from build123d import *

# Parameters (mm, degrees)
F1_DEPTH = 46
F2_R     = 1
F3_DEPTH = 20.001
F5_D     = 4


with BuildPart() as f1:
    # F0 (on Front) → F1 (new body)
    with BuildSketch(Plane.XZ):
        Polygon((33, 0), (0, 0), (0, -20), (7, -20), (7, -7), (33, -7), align=None)
    extrude(amount=F1_DEPTH)

    # F2 (on face) → F3 (cut, through all)
    with BuildSketch(Plane.XY):
        with Locations((24, -4.5)):
            Circle(F2_R)
        with Locations((24, -41.5)):
            Circle(F2_R)
    extrude(amount=-F3_DEPTH, mode=Mode.SUBTRACT)

    # F5 (through all)
    with Locations(Plane.YZ.offset(7)):
        with Locations((-41.5, -13.5), (-4.5, -13.5)):
            Hole(F5_D / 2)


solid = f1.part
Can you work these out from the model? Positions are in its coordinate system, mm. A direction names the side the tool comes from. Coordinates: 2 decimals unless noted, no trailing zeros. Loops run counter-clockwise (first coordinate to the right, second up) from the corner with the lowest first, then second, coordinate; pieces in that order, holes last. Notation, with made-up numbers: M 40,33 L 77,33 A33 cw 77,62 Z; hole C 61,13 d4. An arc over 180 degrees is marked long. Answer as CSV lines item,"result". Start each with the question number.
1. Suppose I cut it at D-D, the plane y = -11.5. List the corners of the cut face in (x, z) for me.
2. For pin 1 Ø8 at (x, y) = (17, -17.5) entering from -Z; pin 2 Ø1 at (y, z) = (-7.5, -17) entering from +X, each with a flat end and sliding along its axis, tell me the tip position at first contact or that it passes through.
3. If I drill on probe 1 along Y at (x, z) = (24, -2); probe 2 along X at (y, z) = (-7.5, -18); probe 3 along Z at (x, y) = (10.5, -26.5), over which ranges is the centre line in solid material (lowest first)? Write a range as [from, to].
4. Suppose I cut it at B-B, the plane x = 24. List the corners of the cut face in (y, z) for me, plus the area to 3 significant figures.
5. Suppose I cut it at A-A, the plane y = -41.5. List the corners of the cut face in (x, z) for me, plus the area to 3 significant figures.
6. Thinking about a two-plate mould opening in Y: for faces 1 (the face through (3.451, -3.026, -12.148)), 2 (the face through (0, -23, -10)), 3 (the face through (13, 0, -5)), 4 (the face through (13, -46, -5)), which applies, +Y half, -Y half, draft (parallel to the pull), parting line (faces both ways), or undercut?
7. Suppose I cut it at C-C, the plane z = -13.5. List the corners of the cut face in (x, y) for me, plus the area to 3 significant figures.
8. For faces 5 (the face through (20, -23, -7)), 6 (the face through (23.263, -3.824, -3.451)), which set-ups out of +Z, -Z, +X, -X, +Y, -Y let a thin tool reach every point of the face, with its end or its side?
Output:
1,outline,"M 0,-20 L 7,-20 L 7,-7 L 33,-7 L 33,0 L 0,0 Z"
2,pin 1,"stops at z = -7"
2,pin 2,"stops at x = 7"
3,probe 1,"y = [-46, -42.5], [-40.5, -5.5], [-3.5, 0]"
3,probe 2,"x = [0, 7]"
3,probe 3,"z = [-7, 0]"
4,outline,"M -46,-7 L -42.5,-7 L -42.5,0 L -46,0 Z; M -40.5,-7 L -5.5,-7 L -5.5,0 L -40.5,0 Z; M -3.5,-7 L 0,-7 L 0,0 L -3.5,0 Z"
4,area,"294 mm^2"
5,outline,"M 0,-20 L 7,-20 L 7,-15.5 L 0,-15.5 Z; M 0,-11.5 L 7,-11.5 L 7,-7 L 23,-7 L 23,0 L 0,0 Z; M 25,-7 L 33,-7 L 33,0 L 25,0 Z"
5,area,"280 mm^2"
6,face 1,"undercut"
6,face 2,"draft"
6,face 3,"+Y half"
6,face 4,"-Y half"
7,outline,"M 0,-46 L 7,-46 L 7,-43.5 L 0,-43.5 Z; M 0,-39.5 L 7,-39.5 L 7,-6.5 L 0,-6.5 Z; M 0,-2.5 L 7,-2.5 L 7,0 L 0,0 Z"
7,area,"266 mm^2"
8,face 5,"-Z, +X, +Y, -Y"
8,face 6,"+Z, -Z"
